```python
from build123d import *

# Parameters (mm, degrees)
CROQUIS1_W              = 45
CROQUIS1_H              = 45
SALIENTE_EXTRUIR1_DEPTH = 25
CROQUIS2_W              = 33
CROQUIS2_H              = 33
CORTAR_EXTRUIR1_DEPTH   = 20
CROQUIS3_R              = 6
CORTAR_EXTRUIR2_DEPTH   = 3
CROQUIS4_R              = 3
CORTAR_EXTRUIR3_DEPTH   = 6
CROQUIS5_R              = 1.75
CORTAR_EXTRUIR4_DEPTH   = 56
CORTAR_EXTRUIR5_DEPTH   = 2
CORTAR_EXTRUIR6_DEPTH   = 2
REDONDEO1_R             = 5
REDONDEO2_R             = 5


with BuildPart() as part:
    # Croquis1 → Saliente-Extruir1 (new body)
    with BuildSketch(Plane.XY):
        Rectangle(CROQUIS1_W, CROQUIS1_H)
    extrude(amount=SALIENTE_EXTRUIR1_DEPTH)

    # Croquis2 → Cortar-Extruir1 (cut)
    with BuildSketch(Plane(origin=(0, 0, 0), x_dir=(-1, 0, 0), z_dir=(0, 0, -1))):
        Rectangle(CROQUIS2_W, CROQUIS2_H)
    extrude(amount=-CORTAR_EXTRUIR1_DEPTH, mode=Mode.SUBTRACT)

    # Croquis3 → Cortar-Extruir2 (cut)
    with BuildSketch(Plane(origin=(0, 0, 20), x_dir=(-1, 0, 0), z_dir=(0, 0, -1))):
        Circle(CROQUIS3_R)
    extrude(amount=-CORTAR_EXTRUIR2_DEPTH, mode=Mode.SUBTRACT)

    # Croquis4 → Cortar-Extruir3 (cut)
    with BuildSketch(Plane(origin=(0, 0, 20), x_dir=(-1, 0, 0), z_dir=(0, 0, -1))):
        Circle(CROQUIS4_R)
    extrude(amount=-CORTAR_EXTRUIR3_DEPTH, mode=Mode.SUBTRACT)

    # Croquis5 → Cortar-Extruir4 (cut)
    with BuildSketch(Plane(origin=(22.5, 0, 0), x_dir=(0, 0, -1), z_dir=(1, 0, 0))):
        with Locations(Location((-6, 0, 0), (0, 0, 90))):
            Circle(CROQUIS5_R)
    extrude(amount=-CORTAR_EXTRUIR4_DEPTH, mode=Mode.SUBTRACT)

    # Croquis6 → Cortar-Extruir5 (cut)
    with BuildSketch(Plane.ZY.offset(-16.5)):
        Polygon((7.962990915, -3.4), (9.92598183, 0), (7.962990915, 3.4), (4.037009085, 3.4), (2.07401817, 0), (4.037009085, -3.4), align=None)
    extrude(amount=-CORTAR_EXTRUIR5_DEPTH, mode=Mode.SUBTRACT)

    # Croquis7 → Cortar-Extruir6 (cut)
    with BuildSketch(Plane(origin=(-16.5, 0, 0), x_dir=(0, 0, -1), z_dir=(1, 0, 0))):
        Polygon((-2.07401817, 0), (-4.037009085, 3.4), (-7.962990915, 3.4), (-9.92598183, 0), (-7.962990915, -3.4), (-4.037009085, -3.4), align=None)
    extrude(amount=-CORTAR_EXTRUIR6_DEPTH, mode=Mode.SUBTRACT)

    # Redondeo1
    redondeo1_edges = [part.edges().sort_by_distance(p)[0] for p in [
        (-16.5, 16.5, 10),
        (-16.5, -16.5, 10),
        (16.5, -16.5, 10),
        (16.5, 16.5, 10),
        (22.5, -22.5, 12.5),
        (-22.5, -22.5, 12.5),
        (-22.5, 22.5, 12.5),
        (22.5, 22.5, 12.5),
    ]]
    fillet(redondeo1_edges, radius=REDONDEO1_R)

    # Redondeo2
    redondeo2_edges = [part.edges().sort_by_distance(p)[0] for p in [
        (0, 22.5, 25),
        (22.5, 0, 25),
        (0, -22.5, 25),
        (21.035533906, 21.035533906, 25),
        (21.035533906, -21.035533906, 25),
        (-21.035533906, -21.035533906, 25),
        (-21.035533906, 21.035533906, 25),
        (-22.5, 0, 25),
    ]]
    fillet(redondeo2_edges, radius=REDONDEO2_R)


solid = part.part
```
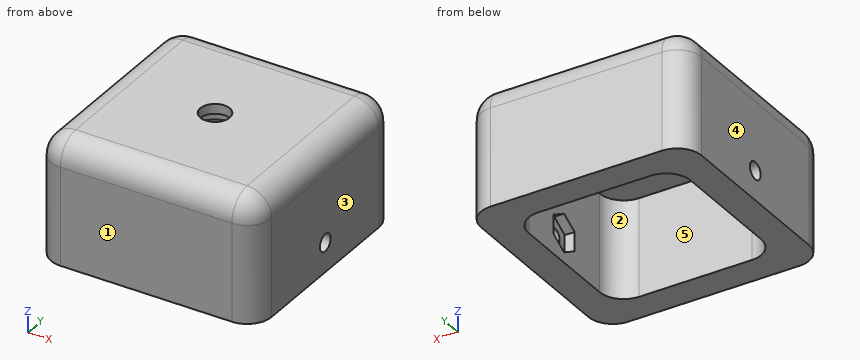
Verification items for the finished model (mm, model axes). Face numbers are marked on the shaded views. A direction names the side the tool comes from. Give positions to 0.01 mm unless a question says otherwise; leave off trailing zeros. Loops run counter-clockwise (first coordinate to the right, second up) from the corner with the lowest first, then second, coordinate; pieces in that order, holes last.
1. Section check C-C, the plane y = -9. Enter the section's corners in (x, z), then the cut area to 3 significant figures.
2. Thickness scan on line 1 (X direction, y = -6, z = 2); line 2 (Y direction, x = 17, z = 4.5). Record the ranges inside material, lowest first.
3. Section check A-A, the plane x = 0. Enter the section's corners in (y, z), then the cut area to 3 significant figures.
4. Go/stop test with flat-tipped pins: pin 1 Ø3 at (y, z) = (0, 6) entering from +X; pin 2 Ø16.5 at (x, y) = (0, -4) entering from -Z; pin 3 Ø7.5 at (y, z) = (0.5, 5) entering from -X; pin 4 Ø9.5 at (x, y) = (0, 0) entering from -Z. Record where each tip stops, or that it passes through.
5. Section check D-D, the plane z = 18. Enter the section's corners in (x, y).
6. Set-up check for the marked faces 4 and 5: record each of +Z, -Z, +X, -X, +Y, -Y from which the full face is reachable in a straight line by a thin tool's end or side.
7. Mould release check, pull along X, two halves, no side actions. Record for the marked faces 1, 2 and 3: released by +X, released by -X, zero draft, split by the parting line, or undercut.
Geometry says:
1. outline: (-22.5, 0) - (-16.5, 0) - (-16.5, 20) - (16.5, 20) - (16.5, 0) - (22.5, 0) - (22.5, 20) arc R5 ccw to (17.5, 25) - (-17.5, 25) arc R5 ccw to (-22.5, 20) - close
1. area: 454 mm2
2. line 1: x = -22.5 to -16.5, 16.5 to 22.5
2. line 2: y = -22.5 to -3.4, 3.4 to 22.5
3. outline: (-22.5, 0) - (-16.5, 0) - (-16.5, 20) - (-6, 20) - (-6, 23) - (-3, 23) - (-3, 25) - (-17.5, 25) arc R5 ccw to (-22.5, 20) - close; (3, 23) - (6, 23) - (6, 20) - (16.5, 20) - (16.5, 0) - (22.5, 0) - (22.5, 20) arc R5 ccw to (17.5, 25) - (3, 25) - close
3. area: 406 mm2
4. pin 1: passes through
4. pin 2: stops at z = 20
4. pin 3: stops at x = -22.5
4. pin 4: stops at z = 23
5. outline: (-22.5, -17.5) arc R5 ccw to (-17.5, -22.5) - (17.5, -22.5) arc R5 ccw to (22.5, -17.5) - (22.5, 17.5) arc R5 ccw to (17.5, 22.5) - (-17.5, 22.5) arc R5 ccw to (-22.5, 17.5) - close; hole (-16.5, -11.5) arc R5 ccw to (-11.5, -16.5) - (11.5, -16.5) arc R5 ccw to (16.5, -11.5) - (16.5, 11.5) arc R5 ccw to (11.5, 16.5) - (-11.5, 16.5) arc R5 ccw to (-16.5, 11.5) - close
6. face 4: +Z, -Z, -X, +Y, -Y
6. face 5: -Z
7. face 1: zero draft
7. face 2: undercut
7. face 3: released by +X
